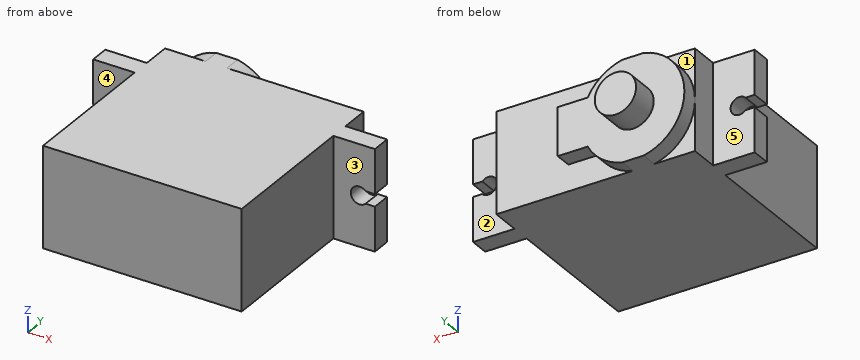
from build123d import *

# Parameters (mm, degrees)
SKETCH1_W           = 22.606
SKETCH1_H           = 11.43
BOSS_EXTRUDE1_DEPTH = 21.971
BOSS_EXTRUDE2_DEPTH = 2.1844
BOSS_EXTRUDE3_DEPTH = 1.905
SKETCH5_R           = 2.3495
BOSS_EXTRUDE4_DEPTH = 3.175


with BuildPart() as part:
    # Sketch1 → Boss-Extrude1 (new body)
    with BuildSketch(Plane(origin=(0, 0, 0), x_dir=(1, 0, 0), z_dir=(0, 1, 0))):
        with Locations((11.303, 5.715)):
            Rectangle(SKETCH1_W, SKETCH1_H)
    extrude(amount=BOSS_EXTRUDE1_DEPTH)

    # Sketch3 → Boss-Extrude2 (add)
    with BuildSketch(Plane(origin=(0, 16.51, 0), x_dir=(1, 0, 0), z_dir=(0, 1, 0))):
        with BuildLine():
            Line((0, 0), (-4.7244, 0))
            Line((-4.7244, 0), (-4.7244, 5.0165))
            Line((-4.7244, 5.0165), (-3.674214486, 5.0165))
            ThreePointArc((-3.674214486, 5.0165), (-1.9812, 5.715), (-3.674214486, 6.4135))
            Line((-3.674214486, 6.4135), (-4.7244, 6.4135))
            Line((-4.7244, 6.4135), (-4.7244, 11.43))
            Line((-4.7244, 11.43), (0, 11.43))
            Line((0, 11.43), (0, 0))
        make_face()
    boss_extrude2 = extrude(amount=BOSS_EXTRUDE2_DEPTH)

    # Sketch4 → Boss-Extrude3 (add)
    with BuildSketch(Plane(origin=(0, 21.971, 0), x_dir=(1, 0, 0), z_dir=(0, 1, 0))):
        with BuildLine():
            Line((4.630497214, 11.43), (7.053502786, 11.43))
            ThreePointArc((7.053502786, 11.43), (9.362022159, 10.377446568), (11.006623292, 8.4455))
            Line((11.006623292, 8.4455), (14.4145, 8.4455))
            Line((14.4145, 8.4455), (14.4145, 2.9845))
            Line((14.4145, 2.9845), (11.006623292, 2.9845))
            ThreePointArc((11.006623292, 2.9845), (9.362022159, 1.052553432), (7.053502786, 0))
            Line((7.053502786, 0), (4.630497214, 0))
            ThreePointArc((4.630497214, 0), (0, 5.715), (4.630497214, 11.43))
        make_face()
    extrude(amount=BOSS_EXTRUDE3_DEPTH)

    # Sketch5 → Boss-Extrude4 (add)
    with BuildSketch(Plane(origin=(0, 23.876, 0), x_dir=(1, 0, 0), z_dir=(0, 1, 0))):
        with Locations(Location((5.842, 5.715, 0), (0, 0, 270))):
            Circle(SKETCH5_R)
    extrude(amount=BOSS_EXTRUDE4_DEPTH)

    # Mirror1: Boss-Extrude2 across plane
    add(boss_extrude2.mirror(Plane(origin=(11.303, 0, 0), x_dir=(0, 0, 1), z_dir=(1, 0, 0))))


solid = part.part
CAD build for the part. Positions are in the model's coordinates, mm. Face numbers are marked on the shaded views. A direction names the side the tool comes from. Round coordinates to 2 decimals unless told otherwise and drop trailing zeros. Order: outer loops, then holes, each group sorted by start corner. A loop starts at its lowest first (then second) coordinate and runs counter-clockwise, first axis right, second up. Notation, with made-up numbers: (33.5, 63) - (82.5, 63) arc R7 cw to (82.5, 72) - close; hole circle Ø8 at (-18, 71). An arc over 180 degrees is marked (long way). Return JSON: item names as keys, results as strings.
(1) Cut at D-D (x = 15.5). Give the cut face in (y, z).
Answer key:
{"outline": "(0, -11.43) - (21.97, -11.43) - (21.97, 0) - (0, 0) - close"}
(2) Tool access for the marked faces 1, 2, 3, 4 and 5: list every direction of +Z, -Z, +X, -X, +Y, -Y with a clear straight run to the whole face (end or side of a thin tool).
Answer key:
{"face 1": "+Z, -X, +Y", "face 2": "+Z, -Z, +X, +Y", "face 3": "+Z, -Z, +X, -Y", "face 4": "+Z, -Z, -X, -Y", "face 5": "+Z, -Z, -X, +Y"}
(3) Cut at A-A (y = 23.25). Give the cut face in (x, z) (1 decimal), then the cut area to 3 significant figures.
Answer key:
{"outline": "(4.6, -11.4) - (7.1, -11.4) arc R5.8 ccw to (11, -8.4) - (14.4, -8.4) - (14.4, -3) - (11, -3) arc R5.8 ccw to (7.1, 0) - (4.6, 0) arc R5.8 ccw to start", "area": "123 mm^2"}
(4) Wall check: probe 1 along X at (y, z) = (9, -8.5); probe 2 along Y at (x, z) = (7.5, -0.75); probe 3 along Y at (x, z) = (24.5, -1.25). Give the ranges that are in metal, low to high. Write a range as from..to.
Answer key:
{"probe 1": "x = 0..22.61", "probe 2": "y = 0..23.88", "probe 3": "y = 16.51..18.69"}
(5) Pin check, flat tips, straight feed: pin 1 Ø1.6 at (x, z) = (25.58, -5.72) entering from +Y; pin 2 Ø2 at (x, y) = (19, 5.5) entering from +Z; pin 3 Ø1.4 at (x, z) = (-1.5, -6) entering from +Y; pin 4 Ø3.5 at (x, z) = (12.5, -5.5) entering from +Y. Stop position of each tip, or through.
Answer key:
{"pin 1": "passes through", "pin 2": "stops at z = 0", "pin 3": "stops at y = 18.69", "pin 4": "stops at y = 23.88"}
(6) Cut at C-C (z = -2.25). Give the cut face in (x, y).
Answer key:
{"outline": "(-4.72, 16.51) - (0, 16.51) - (0, 0) - (22.61, 0) - (22.61, 16.51) - (27.33, 16.51) - (27.33, 18.69) - (22.61, 18.69) - (22.61, 21.97) - (10.55, 21.97) - (10.55, 23.88) - (1.14, 23.88) - (1.14, 21.97) - (0, 21.97) - (0, 18.69) - (-4.72, 18.69) - close"}
(7) Cut at B-B (x = 25.5). Give the cut face in (y, z), then the cut area to 3 significant figures.
Answer key:
{"outline": "(16.51, -11.43) - (18.69, -11.43) - (18.69, -6.7) - (16.51, -6.7) - close; (16.51, -4.73) - (18.69, -4.73) - (18.69, 0) - (16.51, 0) - close", "area": "20.7 mm^2"}
